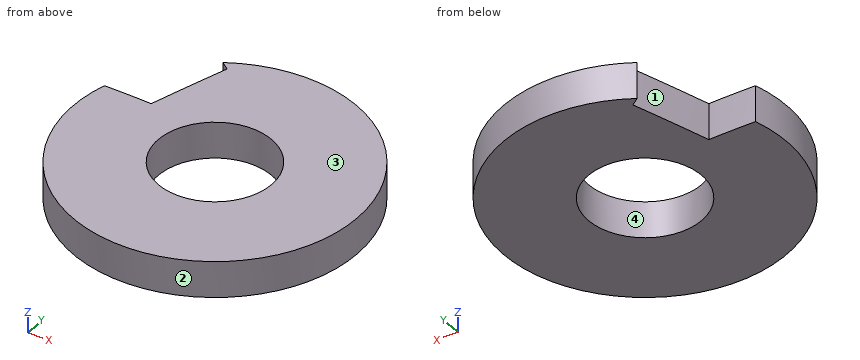
Autodesk Inventor part; units mm, degrees
ref_plane "YZ Plane" through (0, 0, 0) normal (1, 0, 0) x (0, 1, 0)
ref_plane "XZ Plane" through (0, 0, 0) normal (0, 1, 0) x (-1, 0, 0)
ref_plane "XY Plane" through (0, 0, 0) normal (0, 0, 1) x (1, 0, 0)
sketch "Sketch1" plane through (0, 0, 0) normal (0, 0, 1) x (1, 0, 0)
  circle A0 centre (0, 0) radius 7.9375
  circle A1 centre (0, 0) radius 3.175
  dimension "d0" = 15.875
  dimension "d1" = 6.35
extrude "Extrusion1" add sketch "Sketch1" along normal blind 2.032
sketch "Sketch2" plane through (0, 0, 2.032) normal (0, 0, 1) x (1, 0, 0)
  circle A0 centre (0, 0) radius 7.9375 construction
  arc A1 (-5.0493, 2.1833) -> (-17.7625, 1.0248) centre (-5.5945, -62.1721) ccw
  arc A2 (-3.7141, 6.4391) -> (-5.0493, 2.1833) centre (163.5858, -48.389) ccw
  arc A3 (-13.4868, 14.6525) -> (-3.7141, 6.4391) centre (32.6027, 59.5711) ccw
  arc A4 (-4.1702, 6.7537) -> (-7.6399, 2.1531) centre (0, 0) ccw
extrude "Extrusion2" cut sketch "Sketch2" against normal blind 25.4
properties part number "Gear Washer Spacer 4" material "Steel"
The listing builds one solid part. Answer for the finished solid, in the listing's coordinates (mm). Face numbers are marked on the shaded views. Round coordinates to 2 decimals unless told otherwise and drop trailing zeros. Write each loop counter-clockwise with the first axis right and the second up, starting at its lowest first coordinate (ties: lowest second). Pieces come first, ordered by that corner, then holes. Notation, with made-up numbers: M 44.25,-38.75 L 79.25,-38.75 A37 cw 79.25,-2.75 Z; hole C 6.25,16.25 d9. An arc over 180 degrees is marked long. Write each question's results on one line, items separated by ' | '. Start each with the question number.
Item 1: Straight lines are drawn through the part: L1, parallel to Y at x = 0, z = 1.65 (1 decimal); L2, parallel to Y at x = 1.75, z = 0.5; L3, parallel to X at y = 2, z = 1.35. For each, find the intervals that lie inside material, in ascending order. Write a range as [from, to].
Item 2: A cutting plane is placed at A-A on x = 0. Write down the section's boundary in (y, z) (1 decimal).
Item 3: For a pull along Y with two mould halves and no side action, classify the marked faces 1, 2, 3 and 4 as pulls with the +Y half, pulls with the -Y half, needs draft (parallel to the pull), parting line crosses it, or undercut.
Item 4: A cutting plane is placed at D-D on x = -3.5. Write down the section's boundary in (y, z), and give its area (3 significant figures).
Check sheet entries:
1) L1: [-7.9, -3.2], [3.2, 7.9] | L2: [-7.74, -2.65], [2.65, 7.74] | L3: [-7.68, -2.47], [2.47, 7.68]
2) outline: M -7.9,0 L -3.2,0 L -3.2,2 L -7.9,2 Z; M 3.2,0 L 7.9,0 L 7.9,2 L 3.2,2 Z
3) face 1: undercut | face 2: parting line crosses it | face 3: needs draft | face 4: undercut
4) outline: M -7.12,0 L 7.12,0 L 7.12,2.03 L -7.12,2.03 Z | area: 29.0 mm²
